Verification items for the finished model (mm, model axes). A direction names the side the tool comes from. Round coordinates to 2 decimals unless told otherwise and drop trailing zeros. Order: outer loops, then holes, each group sorted by start corner. A loop starts at its lowest first (then second) coordinate and runs counter-clockwise, first axis right, second up.
```python
from build123d import *

# Parameters (mm, degrees)
ESBO_O1_R                  = 175
RESSALTO_EXTRUS_O1_DEPTH   = 20
ESBO_O3_R                  = 175
ESBO_O3_R_2                = 155
RESSALTO_EXTRUS_O3_DEPTH   = 130
ESBO_O4_R                  = 25
CORTE_EXTRUS_O1_DEPTH      = 131
CORTE_EXTRUS_O1_DEPTH_BACK = 21
ESBO_O5_R                  = 30
ESBO_O5_R_2                = 25
RESSALTO_EXTRUS_O4_DEPTH   = 130


with BuildPart() as part:
    # Esboço1 → Ressalto-extrusão1 (new body)
    with BuildSketch(Plane(origin=(0, 0, 0), x_dir=(1, 0, 0), z_dir=(0, 1, 0))):
        Circle(ESBO_O1_R)
    extrude(amount=RESSALTO_EXTRUS_O1_DEPTH)

    # Esboço3 → Ressalto-extrusão3 (add)
    with BuildSketch(Plane(origin=(0, 20, 0), x_dir=(1, 0, 0), z_dir=(0, 1, 0))):
        Circle(ESBO_O3_R)
        Circle(ESBO_O3_R_2, mode=Mode.SUBTRACT)
    extrude(amount=RESSALTO_EXTRUS_O3_DEPTH)

    # Esboço4 → Corte-extrusão1 (cut, two sides)
    with BuildSketch(Plane(origin=(0, 20, 0), x_dir=(1, 0, 0), z_dir=(0, 1, 0))) as corte_extrus_o1_sk:
        Circle(ESBO_O4_R)
    extrude(amount=CORTE_EXTRUS_O1_DEPTH, mode=Mode.SUBTRACT)
    extrude(corte_extrus_o1_sk.sketch, amount=-CORTE_EXTRUS_O1_DEPTH_BACK, mode=Mode.SUBTRACT)

    # Esboço5 → Ressalto-extrusão4 (add, through all)
    with BuildSketch(Plane(origin=(0, 20, 0), x_dir=(1, 0, 0), z_dir=(0, 1, 0))):
        Circle(ESBO_O5_R)
        Circle(ESBO_O5_R_2, mode=Mode.SUBTRACT)
    extrude(amount=RESSALTO_EXTRUS_O4_DEPTH)


solid = part.part
```
1) Sectioned sample at C-C on y = 58.5. Record the cut outline in (x, z).
2) Sectioned sample at A-A on x = 0. Record the cut outline in (y, z).
3) Draft check along Z on faces 1 (the cylindrical face through (-128.982, 73.95, -118.273)), 2 (the flat face through (-14, 150, 155)), 3 (the cylindrical face through (-33.601, 84.09, 151.314)). Enter one of: released by +Z, released by -Z, zero draft, split by the parting line, or undercut.
4) Tool access check on faces 4 (the flat face through (-2, 20, 32)), 5 (the flat face through (-7, 150, -25)). Record the directions out of +Z, -Z, +X, -X, +Y, -Y that give a thin tool (end or side, any length) a straight path to the whole face; none if there is none.
5) Sectioned sample at D-D on x = 71. Record the cut outline in (y, z), then the cut area to 3 significant figures.
6) Sectioned sample at B-B on z = 0. Record the cut outline in (x, y).
7) Scan lines: probe 1 along Z at (x, y) = (0, 55); probe 2 along Z at (x, y) = (0, 5.25). Record each from-to range of solid material in increasing order.
8) Go/stop test with flat-tipped pins: pin 1 Ø10 at (x, y) = (39.5, 19.5) entering from +Z; pin 2 Ø12 at (x, y) = (104, 71.5) entering from +Z; pin 3 Ø1 at (x, y) = (64, 115.5) entering from +Z. Record where each tip stops, or that it passes through.
Returned:
1. outline: circle Ø350 at (0, 0); circle Ø60 at (0, 0); hole circle Ø310 at (0, 0); hole circle Ø50 at (0, 0)
2. outline: (0, -175) - (150, -175) - (150, -155) - (20, -155) - (20, -30) - (150, -30) - (150, -25) - (0, -25) - close; (0, 25) - (150, 25) - (150, 30) - (20, 30) - (20, 155) - (150, 155) - (150, 175) - (0, 175) - close
3. face 1: split by the parting line
3. face 2: zero draft
3. face 3: undercut
4. face 4: +Y
4. face 5: +Z, -Z, +X, -X, +Y
5. outline: (0, -159.95) - (150, -159.95) - (150, -137.78) - (20, -137.78) - (20, 137.78) - (150, 137.78) - (150, 159.95) - (0, 159.95) - close
5. area: 12,200 mm2
6. outline: (-175, 0) - (-25, 0) - (-25, 150) - (-30, 150) - (-30, 20) - (-155, 20) - (-155, 150) - (-175, 150) - close; (25, 0) - (175, 0) - (175, 150) - (155, 150) - (155, 20) - (30, 20) - (30, 150) - (25, 150) - close
7. probe 1: z = -175 to -155, -30 to -25, 25 to 30, 155 to 175
7. probe 2: z = -175 to -25, 25 to 175
8. pin 1: stops at z = 171.57
8. pin 2: stops at z = 144.99
8. pin 3: stops at z = 163.07
